Build history of the part. All positions in model axes, mm. Face numbers are marked on the shaded views. A direction names the side the tool comes from. Give positions to 0.01 mm unless a question says otherwise; leave off trailing zeros. Loops run counter-clockwise (first coordinate to the right, second up) from the corner with the lowest first, then second, coordinate; pieces in that order, holes last. Notation, with made-up numbers: M 15.25,66 L 24.25,66 A24 ccw 24.25,103 Z; hole C 70,35 d6. An arc over 180 degrees is marked long. Answer as a JSON object with one key per item and string values. Group by question number.
1. Drill centre lines: line 1 along X through (y, z) = (-23, -22); line 2 along Z through (x, y) = (-27, -14.5); line 3 along Z through (x, y) = (149.5, -10). Where is each one in solid material? Low to high. Write a range as [from, to].
2. Drop flat-ended pins along their axis: pin 1 Ø5 at (y, z) = (-13, 64) entering from +X; pin 2 Ø7.5 at (x, y) = (-16, -10.5) entering from +Z; pin 3 Ø5 at (x, y) = (115, -5) entering from -Z. Give the stop position or say it passes through.
3. Slice it at B-B (z = 1). List the corners of the cut face in (x, y), then the cut area to 3 significant figures.
4. Slice it at C-C (x = -7). List the corners of the cut face in (y, z).
5. Slice it at A-A (y = -5.25). List the corners of the cut face in (x, z).
6. 3-axis set-ups, long thin cutter, end or side, ignore diameter. For the marked faces 1, 2 and 3: which of +Z, -Z, +X, -X, +Y, -Y reach the whole face in a straight line?
from build123d import *

# Parameters (mm, degrees)
F1_DEPTH = 25.4


with BuildPart() as f1:
    # F0 (on Front) → F1 (new body)
    with BuildSketch(Plane.XZ):
        Polygon((0, 40.874757), (60.281143, 40.874757), (190.667018, 126.703754), (90.644978, 114.797905), align=None)
        Polygon((-60.281143, -40.874757), (60.281143, -40.874757), (60.281143, 40.874757), (0, 40.874757), (-60.281143, 40.874757), align=None)
    extrude(amount=F1_DEPTH)


solid = f1.part
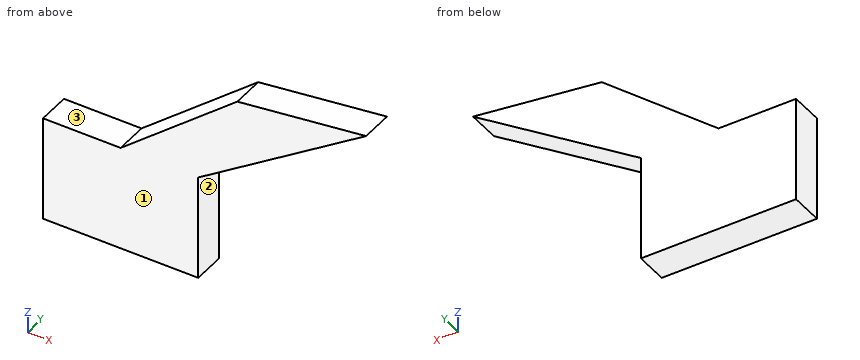
Established:
{
 "1": {"line 1": "x = [-60.28, 60.28]", "line 2": "z = [-40.87, 40.87]", "line 3": "z = [99.6, 121.8]"},
 "2": {"pin 1": "stops at x = 99.21", "pin 2": "stops at z = 40.87", "pin 3": "stops at z = 75.25"},
 "3": {"outline": "M -60.28,-25.4 L 60.28,-25.4 L 60.28,0 L -60.28,0 Z", "area": "3,060 mm^2"},
 "4": {"outline": "M -25.4,-40.87 L 0,-40.87 L 0,40.87 L -25.4,40.87 Z"},
 "5": {"outline": "M -60.28,-40.87 L 60.28,-40.87 L 60.28,40.87 L 190.67,126.7 L 90.64,114.8 L 0,40.87 L -60.28,40.87 Z"},
 "6": {"face 1": "+Z, -Z, +X, -X, -Y", "face 2": "-Z, +X, +Y, -Y", "face 3": "+Z, -X, +Y, -Y"}
}
